Check sheet for the modelled part. Datum: model origin and axes. Units: mm. A direction names the side the tool comes from. Round coordinates to 2 decimals unless told otherwise and drop trailing zeros. Write each loop counter-clockwise with the first axis right and the second up, starting at its lowest first coordinate (ties: lowest second). Pieces come first, ordered by that corner, then holes. Notation, with made-up numbers: M 52.25,53 L 58.25,53 A25 cw 58.25,78 Z; hole C 73,-13 d11. An arc over 180 degrees is marked long. One line per item, written item: value.
from build123d import *

# Parameters (mm, degrees)
SKETCH1_W                       = 43
SKETCH1_H                       = 32.6
BOSS_EXTRUDE1_DEPTH             = 4.875
SKETCH2_R                       = 4
CUT_EXTRUDE1_DEPTH              = 29.688020148
BOSS_EXTRUDE3_REACH             = 30.688
SKETCH3_W                       = 28
SKETCH3_H                       = 10
BOSS_EXTRUDE3_DIRECTION_2_DEPTH = 20
FILLET1_R                       = 3


with BuildPart() as part:
    # Sketch1 → Boss-Extrude1 (new, symmetric)
    with BuildSketch(Plane.XY):
        Rectangle(SKETCH1_W, SKETCH1_H)
    extrude(amount=BOSS_EXTRUDE1_DEPTH, both=True)

    # Sketch2 → Cut-Extrude1 (cut, through all)
    with BuildSketch(Plane.XY.offset(4.875)):
        with Locations((0, 1.3)):
            Circle(SKETCH2_R)
    extrude(amount=-CUT_EXTRUDE1_DEPTH, mode=Mode.SUBTRACT)

    # Boss-Extrude3: up to this face of the body (flat: up to its plane)
    boss_extrude3_end = Plane(part.part.faces().sort_by_distance((0, -15.760392735, -4.875))[0])
    # Sketch3 → Boss-Extrude3 (add, up to the picked face)
    with BuildSketch(Plane.XY.offset(4.875), mode=Mode.PRIVATE) as boss_extrude3_sk1:
        with Locations((0, -21.3)):
            Rectangle(SKETCH3_W, SKETCH3_H)
    boss_extrude3_tool1 = split(extrude(boss_extrude3_sk1.sketch, amount=-BOSS_EXTRUDE3_REACH, mode=Mode.PRIVATE), bisect_by=boss_extrude3_end, keep=Keep.BOTH, mode=Mode.PRIVATE)
    add(boss_extrude3_tool1.solids().sort_by(Axis((0, -21.3, 4.875), (0, 0, -1)))[0])

    # Sketch3 → Boss-Extrude3 direction 2 (add)
    with BuildSketch(Plane.XY.offset(4.875)):
        with Locations((0, -21.3)):
            Rectangle(SKETCH3_W, SKETCH3_H)
    extrude(amount=BOSS_EXTRUDE3_DIRECTION_2_DEPTH)

    # Fillet1
    fillet1_edges = [part.edges().sort_by_distance(p)[0] for p in [
        (-14, -21.3, -4.875),
        (14, -21.3, -4.875),
        (-14, -21.3, 24.875),
        (14, -21.3, 24.875),
        (21.5, -16.3, 0),
        (-21.5, -16.3, 0),
        (-21.5, 16.3, 0),
        (21.5, 16.3, 0),
    ]]
    fillet(fillet1_edges, radius=FILLET1_R)


solid = part.part
Q1. Sectioned sample at D-D on x = 9. Enter the section's corners in (y, z) (3 decimals), and give its area (3 significant figures).
Completed:
outline: M -26.3,-4.875 L 16.3,-4.875 L 16.3,4.875 L -16.3,4.875 L -16.3,24.875 L -26.3,24.875 Z
area: 615 mm^2
Q2. Sectioned sample at C-C on x = 0. Enter the section's corners in (y, z) (3 decimals).
Completed:
outline: M -26.3,-4.875 L -2.7,-4.875 L -2.7,4.875 L -16.3,4.875 L -16.3,24.875 L -26.3,24.875 Z; M 5.3,-4.875 L 16.3,-4.875 L 16.3,4.875 L 5.3,4.875 Z
Q3. Access from +Z, -Z, +X, -X, +Y, -Y to the whole of each face (thin tool, end or side, straight path). Record for faces 1 (the flat face through (0, -3, 4.875)), 2 (the cylindrical face through (13.145, -21.23, -3.973)), 3 (the flat face through (-14, -21, 10)), 4 (the cylindrical face through (-13.145, -21.23, -3.973)), 5 (the flat face through (14, -21, 10)).
Completed:
face 1: +Z, +X, -X, +Y
face 2: -Z, +X, -Y
face 3: +Z, -Z, -X, -Y
face 4: -Z, -X, -Y
face 5: +Z, -Z, +X, -Y
Q4. Sectioned sample at B-B on y = 1.3. Enter the section's corners in (x, z) (3 decimals).
Completed:
outline: M -21.5,-4.875 L -4,-4.875 L -4,4.875 L -21.5,4.875 Z; M 4,-4.875 L 21.5,-4.875 L 21.5,4.875 L 4,4.875 Z
Q5. Scan lines: line 1 (Y direction, x = 0, z = -0.5); line 2 (Z direction, x = -13.5, y = -8) (3 decimals); line 3 (Y direction, x = -6, z = 18.5). Record each from-to range of solid material in increasing order. Write a range as [from, to].
Completed:
line 1: [-26.3, -2.7], [5.3, 16.3]
line 2: [-4.875, 4.875]
line 3: [-26.3, -16.3]
Q6. Draft check along Y on faces 6 (the cylindrical face through (-20.64, -15.4, 0.07)), 7 (the flat face through (0, -5, -4.875)), 8 (the cylindrical face through (-0.867, -2.605, 0.068)). Enter one of: pulls with the +Y half, pulls with the -Y half, needs draft (parallel to the pull), parting line crosses it, or undercut.
Completed:
face 6: pulls with the -Y half
face 7: needs draft
face 8: undercut
Q7. Depth check by flat-ended pin: P1, Ø8, axis at x = -7.5, z = 21.5, coming from the +Y side; P2, Ø1.5, axis at y = -14.5, z = 19.5, coming from the -X side; P3, Ø5, axis at y = -19, z = 7.5, coming from the +X side; P4, Ø10.5, axis at x = 0, y = 1.3, coming from the +Z side (3 decimals). Enter the tip coordinate at first touch or a pass-through.
Completed:
P1: y = -16.3
P2: through
P3: x = 14
P4: z = 4.875
Q8. Sectioned sample at A-A on z = 3.25. Enter the section's corners in (x, y).
Completed:
outline: M -21.5,-13.3 A3 ccw -18.5,-16.3 L -14,-16.3 L -14,-26.3 L 14,-26.3 L 14,-16.3 L 18.5,-16.3 A3 ccw 21.5,-13.3 L 21.5,13.3 A3 ccw 18.5,16.3 L -18.5,16.3 A3 ccw -21.5,13.3 Z; hole C 0,1.3 d8
